Could you check a few things on this drawing? It's one solid part, dimensions in mm from its lowest x, y, z. A direction names the side the tool comes from. Give positions to 0.01 mm unless a question says otherwise; leave off trailing zeros. Order: outer loops, then holes, each group sorted by start corner. A loop starts at its lowest first (then second) coordinate and runs counter-clockwise, first axis right, second up. Notation, with made-up numbers: M 13,8.5 L 50,8.5 A30 cw 50,40.5 Z; hole C 39.25,38.25 d9. An arc over 180 degrees is marked long. One line per item, written item: value. Start each with the question number.
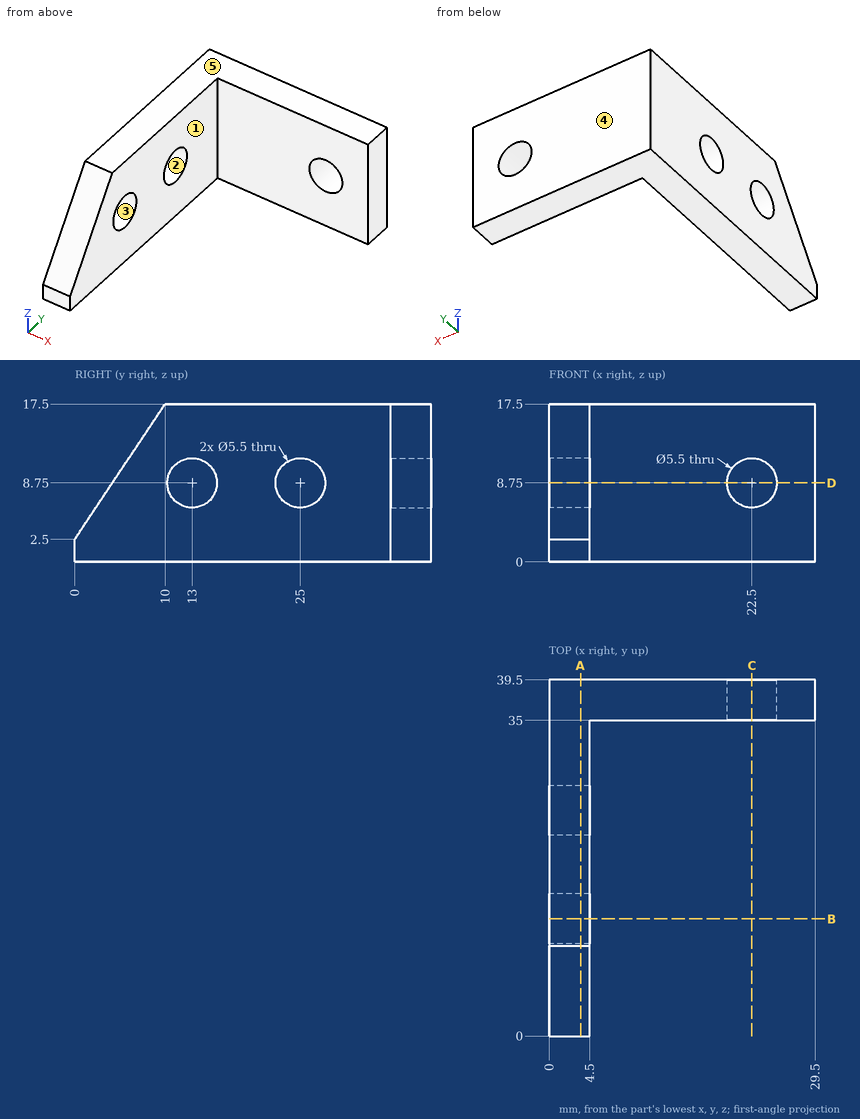
Item 1: Please list where these lines run through material, in increasing order: probe 1 along Z at (x, y) = (22.5, 36.1); probe 2 along X at (y, z) = (23.5, 6.25); probe 3 along Y at (x, z) = (26.5, 5). Write a range as [from, to].
Item 2: Will these pins go through, and if not, where does the flat tip stop? P1, Ø4, axis at x = 4, z = 9, coming from the -Y side; P2, Ø1.5, axis at x = 5.5, z = 10, coming from the -Y side; P3, Ø1.5, axis at y = 30, z = 8.5, coming from the +X side.
Item 3: For the marked faces 1 and 2, which set-ups out of +Z, -Z, +X, -X, +Y, -Y let a thin tool reach every point of the face, with its end or its side?
Item 4: We'd pull the mould along Z, two halves only. Please class the marked faces 3, 4 and 5: +Z half, -Z half, draft (parallel to the pull), parting line (faces both ways), or undercut.
Item 5: I want a section at C-C on x = 22.5. Write out the boundary of the cut face in (y, z), plus the area to 3 significant figures.
Item 6: I want a section at B-B on y = 13. Write out the boundary of the cut face in (x, z).
Item 7: I want a section at A-A on x = 3.5. Write out the boundary of the cut face in (y, z), plus the area to 3 significant figures.
Item 8: I want a section at D-D on z = 8.75. Write out the boundary of the cut face in (x, y).
Answer below:
1. probe 1: z = [0, 6], [11.5, 17.5]
1. probe 2: x = [0, 4.5]
1. probe 3: y = [35, 39.5]
2. P1: stops at y = 3
2. P2: stops at y = 35
2. P3: stops at x = 4.5
3. face 1: +Z, -Z, +X, -Y
3. face 2: +X, -X
4. face 3: undercut
4. face 4: draft
4. face 5: +Z half
5. outline: M 35,0 L 39.5,0 L 39.5,6 L 35,6 Z; M 35,11.5 L 39.5,11.5 L 39.5,17.5 L 35,17.5 Z
5. area: 54.0 mm²
6. outline: M 0,0 L 4.5,0 L 4.5,6 L 0,6 Z; M 0,11.5 L 4.5,11.5 L 4.5,17.5 L 0,17.5 Z
7. outline: M 0,0 L 39.5,0 L 39.5,17.5 L 10,17.5 L 0,2.5 Z; hole C 13,8.75 d5.5; hole C 25,8.75 d5.5
7. area: 569 mm²
8. outline: M 0,4.17 L 4.5,4.17 L 4.5,10.25 L 0,10.25 Z; M 0,15.75 L 4.5,15.75 L 4.5,22.25 L 0,22.25 Z; M 0,27.75 L 4.5,27.75 L 4.5,35 L 19.75,35 L 19.75,39.5 L 0,39.5 Z; M 25.25,35 L 29.5,35 L 29.5,39.5 L 25.25,39.5 Z
